Could you check a few things on this model? Use its own coordinates, in mm. A direction names the side the tool comes from. Round coordinates to 2 decimals unless told otherwise and drop trailing zeros. Order: outer loops, then holes, each group sorted by start corner. A loop starts at its lowest first (then second) coordinate and runs counter-clockwise, first axis right, second up.
```python
from build123d import *

# Parameters (mm, degrees)
BOSS_EXTRUDE1_DEPTH                            = 3
CSK_FOR_M3_FLAT_HEAD_MACHINE_SCREW1_AT_2_COUNT = 2
CSK_FOR_M3_FLAT_HEAD_MACHINE_SCREW1_AT_2_PITCH = 60.801526997
CSK_FOR_M3_FLAT_HEAD_MACHINE_SCREW1_AT_3_COUNT = 2
CSK_FOR_M3_FLAT_HEAD_MACHINE_SCREW1_AT_3_PITCH = 92.34886737
CSK_FOR_M3_FLAT_HEAD_MACHINE_SCREW1_AT_4_COUNT = 2
CSK_FOR_M3_FLAT_HEAD_MACHINE_SCREW1_AT_4_PITCH = 97.558137473
CUT_EXTRUDE1_DEPTH                             = 4
CHAMFER1_SIZE                                  = 0.5


with BuildPart() as part:
    # Sketch2 → Boss-Extrude1 (new body)
    with BuildSketch(Plane.XY.offset(8.62)):
        with BuildLine():
            Line((4.5, 66.2), (95.5, 66.2))
            ThreePointArc((95.5, 66.2), (99.530508653, 64.530508653), (101.2, 60.5))
            Line((101.2, 60.5), (101.2, 26.863961031))
            ThreePointArc((101.2, 26.863961031), (100.766113335, 24.682665466), (99.530508653, 22.833452378))
            Line((99.530508653, 22.833452378), (77.166547622, 0.469491347))
            ThreePointArc((77.166547622, 0.469491347), (75.317334534, -0.766113335), (73.136038969, -1.2))
            Line((73.136038969, -1.2), (4.5, -1.2))
            ThreePointArc((4.5, -1.2), (0.469491347, 0.469491347), (-1.2, 4.5))
            Line((-1.2, 4.5), (-1.2, 60.5))
            ThreePointArc((-1.2, 60.5), (0.469491347, 64.530508653), (4.5, 66.2))
        make_face()
    extrude(amount=BOSS_EXTRUDE1_DEPTH)

    # Sketch5 → CSK for M3 Flat Head Machine Screw1 (revolve, cut)
    with BuildSketch(Plane(origin=(3.085786438, 61.914213562, 11.62), x_dir=(0, -1, 0), z_dir=(1, 0, 0))):
        Polygon((0, 0), (0, 3), (1.7, 3), (1.7, 1.45), (3.15, 0), align=None)
    csk_for_m3_flat_head_machine_screw1 = revolve(axis=Axis((3.085786438, 61.914213562, 17.97), (0, 0, -1)), mode=Mode.SUBTRACT)

    # CSK for M3 Flat Head Machine Screw1 at 2: CSK for M3 Flat Head Machine Screw1 ×2
    with Locations(*[Vector(0.212399494, -0.977182918, 0) * (i * CSK_FOR_M3_FLAT_HEAD_MACHINE_SCREW1_AT_2_PITCH) for i in range(1, CSK_FOR_M3_FLAT_HEAD_MACHINE_SCREW1_AT_2_COUNT)]):
        add(csk_for_m3_flat_head_machine_screw1, mode=Mode.SUBTRACT)

    # CSK for M3 Flat Head Machine Screw1 at 3: CSK for M3 Flat Head Machine Screw1 ×2
    with Locations(*[Vector(0.767001446, -0.641645371, 0) * (i * CSK_FOR_M3_FLAT_HEAD_MACHINE_SCREW1_AT_3_PITCH) for i in range(1, CSK_FOR_M3_FLAT_HEAD_MACHINE_SCREW1_AT_3_COUNT)]):
        add(csk_for_m3_flat_head_machine_screw1, mode=Mode.SUBTRACT)

    # CSK for M3 Flat Head Machine Screw1 at 4: CSK for M3 Flat Head Machine Screw1 ×2
    with Locations(*[Vector(0.962648693, -0.270753565, 0) * (i * CSK_FOR_M3_FLAT_HEAD_MACHINE_SCREW1_AT_4_PITCH) for i in range(1, CSK_FOR_M3_FLAT_HEAD_MACHINE_SCREW1_AT_4_COUNT)]):
        add(csk_for_m3_flat_head_machine_screw1, mode=Mode.SUBTRACT)

    # Sketch6 → Cut-Extrude1 (cut, through all)
    with BuildSketch(Plane.XY.offset(11.62)):
        with BuildLine():
            Line((33.278, 7.9375), (22.483, 7.9375))
            ThreePointArc((22.483, 7.9375), (20.832, 9.5885), (22.483, 11.2395))
            Line((22.483, 11.2395), (33.278, 11.2395))
            ThreePointArc((33.278, 11.2395), (34.929, 9.5885), (33.278, 7.9375))
        make_face()
        with BuildLine():
            Line((33.278, 1.4605), (22.483, 1.4605))
            ThreePointArc((22.483, 1.4605), (20.832, 3.1115), (22.483, 4.7625))
            Line((22.483, 4.7625), (33.278, 4.7625))
            ThreePointArc((33.278, 4.7625), (34.929, 3.1115), (33.278, 1.4605))
        make_face()
        with BuildLine():
            Line((68.326, 1.397), (58.166, 1.397))
            ThreePointArc((58.166, 1.397), (56.515, 3.048), (58.166, 4.699))
            Line((58.166, 4.699), (68.326, 4.699))
            ThreePointArc((68.326, 4.699), (69.977, 3.048), (68.326, 1.397))
        make_face()
    extrude(amount=-CUT_EXTRUDE1_DEPTH, mode=Mode.SUBTRACT)

    # Chamfer1
    chamfer1_edges = [part.edges().sort_by_distance(p)[0] for p in [
        (75.317334534, -0.766113335, 11.62),
        (88.348528137, 11.651471863, 11.62),
        (100.766113335, 24.682665466, 11.62),
        (101.2, 43.681980515, 11.62),
        (99.530508653, 64.530508653, 11.62),
        (50, 66.2, 11.62),
        (0.469491347, 64.530508653, 11.62),
        (-1.2, 32.5, 11.62),
        (0.469491347, 0.469491347, 11.62),
        (34.929, 9.5885, 11.62),
        (27.8805, 11.2395, 11.62),
        (20.832, 9.5885, 11.62),
        (27.8805, 7.9375, 11.62),
        (38.818019485, -1.2, 11.62),
        (34.929, 3.1115, 11.62),
        (27.8805, 4.7625, 11.62),
        (20.832, 3.1115, 11.62),
        (27.8805, 1.4605, 11.62),
        (69.977, 3.048, 11.62),
        (63.246, 4.699, 11.62),
        (56.515, 3.048, 11.62),
        (63.246, 1.397, 11.62),
    ]]
    chamfer(chamfer1_edges, length=CHAMFER1_SIZE)


solid = part.part
```
Q1. Imagine slicing it at B-B, the plane x = 30. Please give me the cut outline in (y, z).
Q2. Imagine slicing it at C-C, the plane z = 9.65. Please give me the cut outline in (x, y), then the cut area to 3 significant figures.
Q3. I need wall thicknesses on L1, parallel to Y at x = 30, z = 9.7; L2, parallel to X at y = 4, z = 10.2; L3, parallel to Y at x = 58, z = 10.4. Which ranges of each line are inside material? Lowest first, please.
Q4. For faces 5 (the flat face through (88.505, 11.808, 9.852)), 6 (the cylindrical face through (20.832, 9.552, 9.888)), 7 (the conical face through (35.064, 9.628, 11.255)), which set-ups out of +Z, -Z, +X, -X, +Y, -Y let a thin tool reach every point of the face, with its end or its side?
Q5. Imagine slicing it at A-A, the plane x = 67. Please give me the cut outline in (y, z).
Q6. We'd pull the mould along Y, two halves only. Please class faces 1 (the conical face through (56.38, 3.009, 11.255)), 2 (the flat face through (49, 66.2, 10)), 3 (the cylindrical face through (17.66, 2.87, 9.41)), 4 (the flat face through (51, 33, 11.62)): released by +Y, released by -Y, zero draft, split by the parting line, or undercut.
Q7. For P1, Ø4, axis at x = 16, y = 2.5, coming from the +Z side, with a flat end and sliding along its axis, tell me the tip position at first contact or that it passes through.
Q8. Imagine slicing it at D-D, the plane x = 16. Please give me the cut outline in (y, z), then the cut area to 3 significant figures.
Filled in:
1. outline: (-1.2, 8.62) - (1.46, 8.62) - (1.46, 11.12) - (0.96, 11.62) - (-0.7, 11.62) - (-1.2, 11.12) - close; (4.76, 8.62) - (7.94, 8.62) - (7.94, 11.12) - (7.44, 11.62) - (5.26, 11.62) - (4.76, 11.12) - close; (11.24, 8.62) - (66.2, 8.62) - (66.2, 11.12) - (65.7, 11.62) - (11.74, 11.62) - (11.24, 11.12) - close
2. outline: (-1.2, 4.5) arc R5.7 ccw to (4.5, -1.2) - (73.14, -1.2) arc R5.7 ccw to (77.17, 0.47) - (99.53, 22.83) arc R5.7 ccw to (101.2, 26.86) - (101.2, 60.5) arc R5.7 ccw to (95.5, 66.2) - (4.5, 66.2) arc R5.7 ccw to (-1.2, 60.5) - close; hole circle Ø3.4 at (3.09, 61.91); hole circle Ø3.4 at (16, 2.5); hole (22.48, 1.46) - (33.28, 1.46) arc R1.65 ccw to (33.28, 4.76) - (22.48, 4.76) arc R1.65 ccw to start; hole (22.48, 7.94) - (33.28, 7.94) arc R1.65 ccw to (33.28, 11.24) - (22.48, 11.24) arc R1.65 ccw to start; hole (58.17, 1.4) - (68.33, 1.4) arc R1.65 ccw to (68.33, 4.7) - (58.17, 4.7) arc R1.65 ccw to start; hole circle Ø3.4 at (73.92, 2.66); hole circle Ø3.4 at (97, 35.5)
2. area: 6,380 mm2
3. L1: y = -1.2 to 1.46, 4.76 to 7.94, 11.24 to 66.2
3. L2: x = -1.18 to 15.14, 16.86 to 21.09, 34.67 to 56.82, 69.67 to 72.82, 75.01 to 80.7
3. L3: y = -1.2 to 1.41, 4.69 to 66.2
4. face 5: +Z, -Z, +X, -Y
4. face 6: +Z, -Z
4. face 7: +Z
5. outline: (-1.2, 8.62) - (1.4, 8.62) - (1.4, 11.12) - (0.9, 11.62) - (-0.7, 11.62) - (-1.2, 11.12) - close; (4.7, 8.62) - (66.2, 8.62) - (66.2, 11.12) - (65.7, 11.62) - (5.2, 11.62) - (4.7, 11.12) - close
6. face 1: undercut
6. face 2: released by +Y
6. face 3: undercut
6. face 4: zero draft
7. P1: stops at z = 10.47
8. outline: (-1.2, 8.62) - (0.8, 8.62) - (0.8, 10.17) - (-0.65, 11.62) - (-0.7, 11.62) - (-1.2, 11.12) - close; (4.2, 8.62) - (66.2, 8.62) - (66.2, 11.12) - (65.7, 11.62) - (5.65, 11.62) - (4.2, 10.17) - close
8. area: 190 mm2
